Source: CAD feature listing. Evaluate the final solid. Frame: model axes, mm. Face numbers are marked on the shaded views. A direction names the side the tool comes from. Give positions to 0.01 mm unless a question says otherwise; leave off trailing zeros. Write each loop counter-clockwise with the first axis right and the second up, starting at its lowest first coordinate (ties: lowest second). Pieces come first, ordered by that corner, then holes. Notation, with made-up numbers: M 37,58 L 47,58 A11 ccw 47,66 Z; hole C 14.25,-15 d6. An arc over 180 degrees is marked long. Use CSV: the item, a comma, the result in double quotes. Start each with the question number.
from build123d import *

# Parameters (mm, degrees)
SKETCHREVOLVEGEARBELT01_W       = 11
SKETCHREVOLVEGEARBELT01_H       = 4.902458105
TOOTHEXTRUDECUTGEARBELT01_DEPTH = 5.5
PATTERNGEARBELT01_COUNT         = 16
SKETCH_5_R                      = 6.5
EXTRUDE_1_DEPTH                 = 1.5
EXTRUDE_START                   = 7
SKETCH_6_R                      = 6.5
EXTRUDE_2_DEPTH                 = 7
CUT_EXTRUDE_2_DEPTH             = 16.516120649
CUT_EXTRUDE_2_DEPTH_BACK        = 16.516120649
SKETCH_7_R                      = 2.5


with BuildPart() as part:
    # SketchRevolveGearBelt01 → GearBelt01 (revolve)
    with BuildSketch(Plane(origin=(0, 0, 0), x_dir=(0, 0, -1), z_dir=(1, 0, 0)), mode=Mode.PRIVATE) as gearbelt01_sk:
        with Locations((0, 2.451229053)):
            Rectangle(SKETCHREVOLVEGEARBELT01_W, SKETCHREVOLVEGEARBELT01_H)
    revolve(gearbelt01_sk.sketch.rotate(Axis((0, 0, 5.5), (0, 0, -1)), 180), axis=Axis((0, 0, 5.5), (0, 0, -1)))

    # SketchToothGearBelt01 → ToothExtrudeCutGearBelt01 (cut, symmetric)
    with BuildSketch(Plane.XY):
        with BuildLine():
            Line((-0.783301597, 4.839476633), (0, 7.442458067))
            Line((0, 7.442458067), (0.783301597, 4.839476633))
            ThreePointArc((0.783301597, 4.839476633), (0.655607945, 4.803813062), (0.599999991, 4.683458109))
            ThreePointArc((0.599999991, 4.683458109), (0, 4.083458118), (-0.599999991, 4.683458109))
            ThreePointArc((-0.599999991, 4.683458109), (-0.655607945, 4.803813062), (-0.783301597, 4.839476633))
        make_face()
    toothextrudecutgearbelt01 = extrude(amount=TOOTHEXTRUDECUTGEARBELT01_DEPTH, both=True, mode=Mode.SUBTRACT)

    # PatternGearBelt01: ToothExtrudeCutGearBelt01 ×16 about axis
    patterngearbelt01_axis = Axis((0, 0, 0), (0, 0, 1))
    for i in range(1, PATTERNGEARBELT01_COUNT):
        add(toothextrudecutgearbelt01.rotate(patterngearbelt01_axis, i * 360 / PATTERNGEARBELT01_COUNT), mode=Mode.SUBTRACT)

    # Sketch 5 → Extrude 1 (add)
    with BuildSketch(Plane.XY.offset(5.5)):
        Circle(SKETCH_5_R)
    extrude(amount=EXTRUDE_1_DEPTH)

    # Sketch 6 → Extrude 2 (add)
    with BuildSketch(Plane(origin=(0, 0, -5.5), x_dir=(-1, 0, 0), z_dir=(0, 0, -1)).offset(EXTRUDE_START)):
        with Locations(Location((0, 0, 0), (0, 0, 180))):
            Circle(SKETCH_6_R)
    extrude(amount=-EXTRUDE_2_DEPTH)

    # Sketch 7 → Cut-Extrude 2 (cut, two sides: drawn at the far end of the back side and taken through both)
    with BuildSketch(Plane.XY.offset(-CUT_EXTRUDE_2_DEPTH_BACK)):
        Circle(SKETCH_7_R)
    extrude(amount=CUT_EXTRUDE_2_DEPTH + CUT_EXTRUDE_2_DEPTH_BACK, mode=Mode.SUBTRACT)


solid = part.part
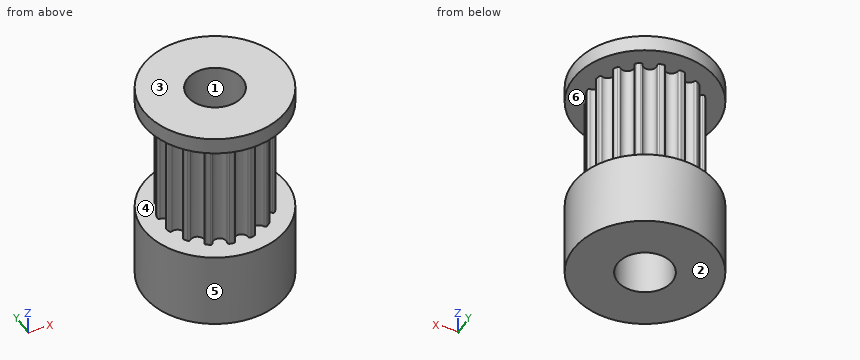
Item 1: Set-up query: the marked faces 5 and 6. Return all of +Z, -Z, +X, -X, +Y, -Y with unobstructed straight access to the full face (end or side cutting, diameter ignored); none if empty.
Item 2: Section D-D (y = -5.5). Return the cut outline in (x, z).
Item 3: Section C-C (z = -6). Return the cut outline in (x, y), plus the area to 3 significant figures.
Item 4: Material intervals for probe 1 along Y at (x, z) = (0, -6.25); probe 2 along Z at (x, y) = (5.25, 3); probe 3 along Y at (x, z) = (0, -3), sorted ascending.
Item 5: Section A-A (x = 0). Return the cut outline in (y, z).
Item 6: Contact query for flat-ended pins moving along their axis: pin 1 Ø3 at (x, z) = (4, -5) entering from +Y; pin 2 Ø2 at (x, z) = (4.5, -3) entering from +Y. Output: stop coordinate, or through.
Item 7: Pull-direction query (Z, two-part tool) for the marked faces 1, 2, 3 and 4; classes: released by +Z, released by -Z, zero draft, split by the parting line, or undercut.
Output values:
1,face 5,"+Z, -Z"
1,face 6,"none"
2,outline,"M -3.46,-12.5 L 3.46,-12.5 L 3.46,-5.5 L -3.46,-5.5 Z; M -3.46,5.5 L 3.46,5.5 L 3.46,7 L -3.46,7 Z"
3,outline,"C 0,0 d13; hole C 0,0 d5"
3,area,"113 mm2"
4,probe 1,"y = -6.5 to -2.5, 2.5 to 6.5"
4,probe 2,"z = -12.5 to -5.5, 5.5 to 7"
4,probe 3,"y = -4.08 to -2.5, 2.5 to 4.08"
5,outline,"M -6.5,-12.5 L -2.5,-12.5 L -2.5,7 L -6.5,7 L -6.5,5.5 L -4.08,5.5 L -4.08,-5.5 L -6.5,-5.5 Z; M 2.5,-12.5 L 6.5,-12.5 L 6.5,-5.5 L 4.08,-5.5 L 4.08,5.5 L 6.5,5.5 L 6.5,7 L 2.5,7 Z"
6,pin 1,"stops at y = 5.96"
6,pin 2,"stops at y = 2.93"
7,face 1,"zero draft"
7,face 2,"released by -Z"
7,face 3,"released by +Z"
7,face 4,"undercut"
